```python
from build123d import *

# Parameters (mm, degrees)
CROQUIS1_R              = 15
CROQUIS1_R_2            = 13
EXTRUIR_L_MINA1_DEPTH   = 18
CROQUIS2_R              = 75
SALIENTE_EXTRUIR1_DEPTH = 8
CROQUIS3_R              = 1.59
CROQUIS3_R_2            = 1.5875
CORTAR_EXTRUIR1_DEPTH   = 10
CROQUIS5_R              = 3.969
CORTAR_EXTRUIR2_DEPTH   = 10
CROQUIS6_R              = 3.5
CORTAR_EXTRUIR3_DEPTH   = 3


with BuildPart() as part:
    # Croquis1 → Extruir-Lámina1 (new body)
    with BuildSketch(Plane(origin=(0, 0, 0), x_dir=(1, 0, 0), z_dir=(0, 1, 0))):
        Circle(CROQUIS1_R)
        Circle(CROQUIS1_R_2, mode=Mode.SUBTRACT)
    extrude(amount=EXTRUIR_L_MINA1_DEPTH)

    # Croquis2 → Saliente-Extruir1 (add)
    with BuildSketch(Plane(origin=(0, 18, 0), x_dir=(1, 0, 0), z_dir=(0, 1, 0))):
        Circle(CROQUIS2_R)
    extrude(amount=SALIENTE_EXTRUIR1_DEPTH)

    # Croquis3 → Cortar-Extruir1 (cut)
    with BuildSketch(Plane(origin=(0, 26, 0), x_dir=(1, 0, 0), z_dir=(0, 1, 0))):
        with Locations((5.896947673, 6.464403154)):
            Circle(CROQUIS3_R)
        with Locations((-5.896947673, -6.464403154)):
            Circle(CROQUIS3_R)
        with Locations((6.492053366, -5.922170706)):
            Circle(CROQUIS3_R)
        with Locations((-6.464403154, 5.896947673)):
            Circle(CROQUIS3_R_2)
    extrude(amount=-CORTAR_EXTRUIR1_DEPTH, mode=Mode.SUBTRACT)

    # Croquis5 → Cortar-Extruir2 (cut)
    with BuildSketch(Plane.XZ.offset(-18)):
        with Locations((0, -63)):
            Circle(CROQUIS5_R)
        with Locations((-63, 0)):
            Circle(CROQUIS5_R)
        with Locations((0, 63)):
            Circle(CROQUIS5_R)
        with Locations((63, 0)):
            Circle(CROQUIS5_R)
    extrude(amount=-CORTAR_EXTRUIR2_DEPTH, mode=Mode.SUBTRACT)

    # Croquis6 → Cortar-Extruir3 (cut)
    with BuildSketch(Plane(origin=(0, 26, 0), x_dir=(1, 0, 0), z_dir=(0, 1, 0))):
        with Locations((5.896947673, 6.464403154)):
            Circle(CROQUIS6_R)
        with Locations((-6.464403154, 5.896947673)):
            Circle(CROQUIS6_R)
        with Locations((-5.896947673, -6.464403154)):
            Circle(CROQUIS6_R)
        with Locations((6.492053366, -5.922170706)):
            Circle(CROQUIS6_R)
    extrude(amount=-CORTAR_EXTRUIR3_DEPTH, mode=Mode.SUBTRACT)


solid = part.part
```
Verification items for the finished model (mm, model axes). A direction names the side the tool comes from. Coordinates: 2 decimals unless noted, no trailing zeros. Order: outer loops, then holes, each group sorted by start corner. A loop starts at its lowest first (then second) coordinate and runs counter-clockwise, first axis right, second up. Notation, with made-up numbers: (34.25, -40) - (67.25, -40) arc R11 cw to (67.25, -20) - close; hole circle Ø1 at (88.25, -28). An arc over 180 degrees is marked (long way). Return JSON: item names as keys, results as strings.
(1) Section check A-A, the plane x = 0. Record the cut outline in (y, z), and give its area (3 significant figures).
Filled sheet:
{"outline": "(0, -15) - (18, -15) - (18, -59.03) - (26, -59.03) - (26, 59.03) - (18, 59.03) - (18, 15) - (0, 15) - (0, 13) - (18, 13) - (18, -13) - (0, -13) - close; (18, -75) - (26, -75) - (26, -66.97) - (18, -66.97) - close; (18, 66.97) - (26, 66.97) - (26, 75) - (18, 75) - close", "area": "1,140 mm^2"}
(2) Go/stop test with flat-tipped pins: pin 1 (6 mm diameter, centred on x = 56, y = 21, fed in from +Z); pin 2 (5 mm diameter, centred on x = 0, z = -63, fed in from +Y); pin 3 (2 mm diameter, centred on x = -5, z = 7.5, fed in from +Y); pin 4 (6.5 mm diameter, centred on x = -5.9, z = 6.46, fed in from -Y). Record where each tip stops, or that it passes through.
Filled sheet:
{"pin 1": "stops at z = 53.07", "pin 2": "passes through", "pin 3": "stops at y = 23", "pin 4": "stops at y = 18"}
(3) Section check D-D, the plane x = -63. Record the cut outline in (y, z), and give its area (3 significant figures).
Filled sheet:
{"outline": "(18, -40.69) - (26, -40.69) - (26, -3.97) - (18, -3.97) - close; (18, 3.97) - (26, 3.97) - (26, 40.69) - (18, 40.69) - close", "area": "588 mm^2"}
(4) Access from +Z, -Z, +X, -X, +Y, -Y to the whole of each face (thin tool, end or side, straight path). Record for faces 5 (the flat face through (-6, 23, -4)), 6 (the cylindrical face through (-14.985, 8.874, -0.66)), 7 (the cylindrical face through (-59.334, 21.944, -1.52)).
Filled sheet:
{"face 5": "+Y", "face 6": "-Y", "face 7": "+Y, -Y"}
(5) Thickness scan on line 1 along Z through (x, y) = (0, 24); line 2 along Y through (x, z) = (0.5, -67); line 3 along X through (y, z) = (1.75, -3.5). Record the ranges inside material, lowest first.
Filled sheet:
{"line 1": "z = -75 to -66.97, -59.03 to 59.03, 66.97 to 75", "line 2": "y = 18 to 26", "line 3": "x = -14.59 to -12.52, 12.52 to 14.59"}
(6) Mould release check, pull along X, two halves, no side actions. Record for faces 1 (the cylindrical face through (9.13, 24.52, -5.12)), 2 (the flat face through (0, 18, 0)), 3 (the flat face through (-1, 26, -1)), 4 (the cylindrical face through (-9.764, 21.944, -74.362)): pulls with the +X half, pulls with the -X half, needs draft (parallel to the pull), parting line crosses it, or undercut.
Filled sheet:
{"face 1": "undercut", "face 2": "undercut", "face 3": "needs draft", "face 4": "parting line crosses it"}
(7) Section check B-B, the plane z = -63. Record the cut outline in (x, y).
Filled sheet:
{"outline": "(-40.69, 18) - (-3.97, 18) - (-3.97, 26) - (-40.69, 26) - close; (3.97, 18) - (40.69, 18) - (40.69, 26) - (3.97, 26) - close"}
(8) Section check C-C, the plane y = 5.75. Record the cut outline in (x, z).
Filled sheet:
{"outline": "circle Ø30 at (0, 0); hole circle Ø26 at (0, 0)"}
